Work out the finished part from the listing and answer in its coordinate system (mm). A direction names the side the tool comes from. Give positions to 0.01 mm unless a question says otherwise; leave off trailing zeros. Loops run counter-clockwise (first coordinate to the right, second up) from the corner with the lowest first, then second, coordinate; pieces in that order, holes last. Notation, with made-up numbers: (-10, 39) - (21, 39) arc R15 ccw to (21, 60) - close; hole circle Ø7 at (-31, 59). An arc over 180 degrees is marked (long way). One line per item, written item: value.
from build123d import *

# Parameters (mm, degrees)
SKETCH1_W                            = 102
SKETCH1_H                            = 26.3
SKETCH1_R                            = 6.15
BASE_DEPTH                           = 20.2
BACKSIDE_SURFACE_1_REACH             = 109.255
SKETCH2_W                            = 60.3
SKETCH2_H                            = 20.3
BACKSIDE_SURFACE_1_DIRECTION_2_DEPTH = 108.255442752
SKETCH4_W                            = 6
SKETCH4_H                            = 26.3
LEG_DEPTH                            = 50
SKETCH5_W                            = 26.3
SKETCH5_H                            = 6
ROOF_DEPTH                           = 102
SKETCH6_R                            = 6.15
HOLE_FOR_LINEAR_ROD_DEPTH            = 26.2
SKETCH9_W                            = 35.7
SKETCH9_H                            = 20
BOSS_EXTRUDE5_DEPTH                  = 26.2
SKETCH7_W                            = 40.3
SKETCH7_H                            = 50
BACKSIDE_SURFACE_2_DEPTH             = 6
BOLT_HOLES_REACH                     = 124.669
SKETCH3_R                            = 2.75
CHAMFER1_SIZE                        = 6
CHAMFER1_SIZE_2                      = 20
FILLET1_R                            = 3


with BuildPart() as part:
    # Sketch1 → base (new body)
    with BuildSketch(Plane(origin=(0, 0, 0), x_dir=(1, 0, 0), z_dir=(0, 1, 0))):
        with Locations((51, 13.15)):
            Rectangle(SKETCH1_W, SKETCH1_H)
        with Locations(Location((87, 10, 0), (0, 0, 270))):
            Circle(SKETCH1_R, mode=Mode.SUBTRACT)
    extrude(amount=BASE_DEPTH)

    # Sketch2 → backside surface 1 (cut, up to next)
    with BuildSketch(Plane(origin=(0, 20.2, 0), x_dir=(1, 0, 0), z_dir=(0, 1, 0)), mode=Mode.PRIVATE) as backside_surface_1_sk1:
        with Locations((30.15, 10.15)):
            Rectangle(SKETCH2_W, SKETCH2_H)
    backside_surface_1_tool1 = extrude(backside_surface_1_sk1.sketch, amount=-BACKSIDE_SURFACE_1_REACH, mode=Mode.PRIVATE) & part.part
    add(backside_surface_1_tool1.solids().sort_by_distance((30.15, 20.2, -10.15))[0], mode=Mode.SUBTRACT)

    # Sketch2 → backside surface 1 direction 2 (cut)
    with BuildSketch(Plane(origin=(0, 20.2, 0), x_dir=(1, 0, 0), z_dir=(0, 1, 0))):
        with Locations((30.15, 10.15)):
            Rectangle(SKETCH2_W, SKETCH2_H)
    extrude(amount=BACKSIDE_SURFACE_1_DIRECTION_2_DEPTH, mode=Mode.SUBTRACT)

    # Sketch4 → leg (add)
    with BuildSketch(Plane(origin=(0, 0, 0), x_dir=(1, 0, 0), z_dir=(0, 1, 0))):
        with Locations((63.3, 13.15)):
            Rectangle(SKETCH4_W, SKETCH4_H)
    extrude(amount=-LEG_DEPTH)

    # Sketch5 → roof (add)
    with BuildSketch(Plane.ZY):
        with Locations((-13.15, 23.2)):
            Rectangle(SKETCH5_W, SKETCH5_H)
    extrude(amount=-ROOF_DEPTH)

    # Sketch6 → hole for linear rod (cut)
    with BuildSketch(Plane.XZ):
        with Locations(Location((87, -10, 0), (0, 0, 90))):
            Circle(SKETCH6_R)
    extrude(amount=-HOLE_FOR_LINEAR_ROD_DEPTH, mode=Mode.SUBTRACT)

    # Sketch9 → Boss-Extrude5 (add)
    with BuildSketch(Plane(origin=(0, 26.2, 0), x_dir=(1, 0, 0), z_dir=(0, 1, 0))):
        with Locations((84.15, -10)):
            Rectangle(SKETCH9_W, SKETCH9_H)
    extrude(amount=-BOSS_EXTRUDE5_DEPTH)

    # Sketch7 → backside surface 2 (add)
    with BuildSketch(Plane.XY.offset(-26.3)):
        with Locations((40.15, -25)):
            Rectangle(SKETCH7_W, SKETCH7_H)
    extrude(amount=BACKSIDE_SURFACE_2_DEPTH)

    # Sketch3 → bolt holes (cut, up to next)
    with BuildSketch(Plane.XY.offset(-26.3), mode=Mode.PRIVATE) as bolt_holes_sk1:
        with Locations((12, 10)):
            Circle(SKETCH3_R)
    bolt_holes_tool1 = extrude(bolt_holes_sk1.sketch, amount=BOLT_HOLES_REACH, mode=Mode.PRIVATE) & part.part
    # Sketch3 → bolt holes (cut, up to next)
    with BuildSketch(Plane.XY.offset(-26.3), mode=Mode.PRIVATE) as bolt_holes_sk2:
        with Locations(Location((52, 10, 0), (0, 0, 180))):
            Circle(SKETCH3_R)
    bolt_holes_tool2 = extrude(bolt_holes_sk2.sketch, amount=BOLT_HOLES_REACH, mode=Mode.PRIVATE) & part.part
    # Sketch3 → bolt holes (cut, up to next)
    with BuildSketch(Plane.XY.offset(-26.3), mode=Mode.PRIVATE) as bolt_holes_sk3:
        with Locations((30, -10)):
            Circle(SKETCH3_R)
    bolt_holes_tool3 = extrude(bolt_holes_sk3.sketch, amount=BOLT_HOLES_REACH, mode=Mode.PRIVATE) & part.part
    # Sketch3 → bolt holes (cut, up to next)
    with BuildSketch(Plane.XY.offset(-26.3), mode=Mode.PRIVATE) as bolt_holes_sk4:
        with Locations((30, -40)):
            Circle(SKETCH3_R)
    bolt_holes_tool4 = extrude(bolt_holes_sk4.sketch, amount=BOLT_HOLES_REACH, mode=Mode.PRIVATE) & part.part
    # Sketch3 → bolt holes (cut, up to next)
    with BuildSketch(Plane.XY.offset(-26.3), mode=Mode.PRIVATE) as bolt_holes_sk5:
        with Locations(Location((50, -40, 0), (0, 0, 180))):
            Circle(SKETCH3_R)
    bolt_holes_tool5 = extrude(bolt_holes_sk5.sketch, amount=BOLT_HOLES_REACH, mode=Mode.PRIVATE) & part.part
    # Sketch3 → bolt holes (cut, up to next)
    with BuildSketch(Plane.XY.offset(-26.3), mode=Mode.PRIVATE) as bolt_holes_sk6:
        with Locations(Location((50, -10, 0), (0, 0, 180))):
            Circle(SKETCH3_R)
    bolt_holes_tool6 = extrude(bolt_holes_sk6.sketch, amount=BOLT_HOLES_REACH, mode=Mode.PRIVATE) & part.part
    add(bolt_holes_tool1.solids().sort_by_distance((12, 10, -26.3))[0], mode=Mode.SUBTRACT)
    add(bolt_holes_tool2.solids().sort_by_distance((52, 10, -26.3))[0], mode=Mode.SUBTRACT)
    add(bolt_holes_tool3.solids().sort_by_distance((30, -10, -26.3))[0], mode=Mode.SUBTRACT)
    add(bolt_holes_tool4.solids().sort_by_distance((30, -40, -26.3))[0], mode=Mode.SUBTRACT)
    add(bolt_holes_tool5.solids().sort_by_distance((50, -40, -26.3))[0], mode=Mode.SUBTRACT)
    add(bolt_holes_tool6.solids().sort_by_distance((50, -10, -26.3))[0], mode=Mode.SUBTRACT)

    # Chamfer1
    # the kernel refuses this chamfer: 20, 6 mm, written as the material it adds along each edge
    with BuildSketch(Plane(origin=(66.3, 26.2, 0), x_dir=(-0.9925205348140392, 0, -0.12207779475585914), z_dir=(0, -1, 0))) as chamfer1_piece_1:
        Polygon((CHAMFER1_SIZE * 0.992520534814, -CHAMFER1_SIZE * 0.122077794756), (-CHAMFER1_SIZE_2 * 0.122077794756, -CHAMFER1_SIZE_2 * 0.992520534814), (0, 0), align=None)
    extrude(amount=26.2)

    # Fillet1
    fillet1_edges = [part.edges().sort_by_distance(p)[0] for p in [
        (30.15, 26.2, 0),
        (63.3, 0, 0),
        (63.3, 26.2, 10),
        (43.15, -50, -26.3),
        (66.3, -50, -13.15),
        (66.3, -25, -26.3),
        (66.3, -25, 0),
        (66.3, 0, -13.15),
        (84.15, 0, -26.3),
        (102, 0, -3.15),
        (51, 26.2, -26.3),
        (0, 23.2, 0),
        (0, 26.2, -13.15),
        (102, 26.2, -3.15),
        (84.15, 26.2, 20),
        (84.15, 0, 20),
        (102, 13.1, 20),
        (66.3, 13.1, 20),
        (0, 13.1, -26.3),
        (102, 13.1, -26.3),
        (10, 0, -26.3),
        (20, -25, -26.3),
    ]]
    fillet(fillet1_edges, radius=FILLET1_R)


solid = part.part
1. Section C-C (x = 88.5) is taken. Write down the section's boundary in (y, z), and give its area (3 significant figures).
Output:
outline: (0, -23.3) arc R3 ccw to (3, -26.3) - (23.2, -26.3) arc R3 ccw to (26.2, -23.3) - (26.2, -15.96) - (0, -15.96) - close; (0, -4.04) - (26.2, -4.04) - (26.2, 17) arc R3 ccw to (23.2, 20) - (3, 20) arc R3 ccw to (0, 17) - close
area: 893 mm²
2. Section A-A (y = 10) is taken. Write down the section's boundary in (x, z), and give its area (3 significant figures).
Output:
outline: (0, -23.3) arc R3 ccw to (3, -26.3) - (9.25, -26.3) - (9.25, -20.3) - (0, -20.3) - close; (14.75, -26.3) - (49.25, -26.3) - (49.25, -20.3) - (14.75, -20.3) - close; (54.75, -26.3) - (99, -26.3) arc R3 ccw to (102, -23.3) - (102, 17) arc R3 ccw to (99, 20) - (68.53, 20) arc R3 ccw to (65.66, 17.86) - (60.3, 0) - (60.3, -20.3) - (54.75, -20.3) - close; hole circle Ø12.3 at (87, -10)
area: 2,040 mm²
3. Find the intervals of material crossed by line 1 along X through (y, z) = (-40, -23.7); line 2 along Y through (x, z) = (30, -21.7); line 3 along Y through (x, z) = (50, -23.4), in increasing order.
Output:
line 1: x = 20.03 to 27.25, 32.75 to 47.25, 52.75 to 66.27
line 2: y = -50 to -42.75, -37.25 to -12.75, -7.25 to 26.2
line 3: y = -50 to -42.75, -37.25 to -12.75, -7.25 to 8.11, 11.89 to 26.2
4. Section B-B (z = -21.5) is taken. Write down the section's boundary in (x, y).
Output:
outline: (0, 0) - (20, 0) - (20, -50) - (63.3, -50) arc R3 ccw to (66.3, -47) - (66.3, -3) arc R3 cw to (69.3, 0) - (99, 0) arc R3 ccw to (102, 3) - (102, 23.2) arc R3 ccw to (99, 26.2) - (3, 26.2) arc R3 ccw to (0, 23.2) - close; hole circle Ø5.5 at (12, 10); hole circle Ø5.5 at (30, -40); hole circle Ø5.5 at (30, -10); hole circle Ø5.5 at (50, -40); hole circle Ø5.5 at (50, -10); hole circle Ø5.5 at (52, 10)
5. The mould has two halves that part along X. Classify faces 6 (the cylindrical face through (54.747, 9.879, -23.342)), 7 (the cylindrical face through (101.1, 25.34, -3.43)), 8 (the cylindrical face through (20.9, -23.13, -25.44)), 9 (the cylindrical face through (82.44, 0.9, 19.14)): released by +X, released by -X, zero draft, split by the parting line, or undercut.
Output:
face 6: undercut
face 7: released by +X
face 8: released by -X
face 9: zero draft
6. Section D-D (y = -10) is taken. Write down the section's boundary in (x, z).
Output:
outline: (20, -23.3) arc R3 ccw to (23, -26.3) - (27.25, -26.3) - (27.25, -20.3) - (20, -20.3) - close; (32.75, -26.3) - (47.25, -26.3) - (47.25, -20.3) - (32.75, -20.3) - close; (52.75, -26.3) - (63.3, -26.3) arc R3 ccw to (66.3, -23.3) - (66.3, -3) arc R3 ccw to (63.3, 0) - (60.3, 0) - (60.3, -20.3) - (52.75, -20.3) - close
7. Flat-ended cylindrical pins translate along their axes: pin 1 Ø4.5 at (x, y) = (52, 10) entering from -Z; pin 2 Ø2.5 at (x, y) = (62.5, -27.5) entering from +Z; pin 3 Ø8 at (y, z) = (-14.5, -20.5) entering from +X; pin 4 Ø6 at (x, y) = (21, -41) entering from -Z. Find the tip coordinate at first contact, or state that the pin passes through.
Output:
pin 1: passes through
pin 2: stops at z = 0
pin 3: stops at x = 66.3
pin 4: stops at z = -26.3
8. For faces 1 (the flat face through (60.3, -14, -10)), 2 (the cylindrical face through (65.4, -26.83, -0.86)), 3 (the flat face through (20, -25, -22)), 4 (the cylindrical face through (33.18, 25.3, -0.86)), 5 (the cylindrical face through (65.4, -25.31, -25.44)), determine the directions among +Z, -Z, +X, -X, +Y, -Y from which every point of the face is accessible in a straight line to the end or side of a thin tool.
Output:
face 1: +Z, -X, -Y
face 2: +Z, +X, -Y
face 3: +Z, -Z, -X, -Y
face 4: +Z, -X, +Y
face 5: -Z, +X, -Y
